The listing builds one solid part. Answer for the finished solid, in the listing's coordinates (mm). Face numbers are marked on the shaded views. A direction names the side the tool comes from. Give positions to 0.01 mm unless a question says otherwise; leave off trailing zeros. Order: outer loops, then holes, each group sorted by start corner. A loop starts at its lowest first (then second) coordinate and runs counter-clockwise, first axis right, second up. Notation, with made-up numbers: (49.25, 48) - (90.25, 48) arc R26 ccw to (90.25, 73) - close; hole circle Ø6 at (42, -1). An arc over 180 degrees is marked (long way). Answer as CSV lines item,"result". Start each with the question number.
1. Section D-D on x = 12.85 is taken. Give the vertices of the cut face in (y, z), and give its area (3 significant figures).
2. Section B-B on x = -20.35 is taken. Give the vertices of the cut face in (y, z).
3. Which of the six approach directions +Z, -Z, +X, -X, +Y, -Y give full straight-line access (tool end or side, diameter ignored) to the marked faces 1 and 2?
4. Flat-ended cylindrical pins translate along their axes: pin 1 (4 mm diameter, centred on x = 20.35, z = -6.35, fed in from -Y); pin 2 (2 mm diameter, centred on x = 10.5, y = -2, fed in from +Z); pin 3 (1.5 mm diameter, centred on y = -2, z = 7.5, fed in from +X). Find the tip coordinate at first contact, or state that the pin passes through.
5. Section C-C on z = -6.35 is taken. Give the vertices of the cut face in (x, y).
6. Consider line 1 along Y through (x, z) = (12.85, -13.55); line 2 along X through (y, z) = (0.9, 9.35); line 3 along Z through (x, y) = (15, -3.25). Determine where each line is inside the solid, lowest interval first. Write a range as [from, to].
7. Section A-A on y = -4 is taken. Give the vertices of the cut face in (x, z), and give its area (3 significant figures).
from build123d import *

# Parameters (mm, degrees)
IZIM1_W                     = 45.7
IZIM1_H                     = 24.3
Y_KSEKLIK_EKSTR_ZYON1_DEPTH = 3
IZIM2_R                     = 1.6
KES_EKSTR_ZYON1_DEPTH       = 21.8
IZIM4_W                     = 45.7
IZIM4_H                     = 2
Y_KSEKLIK_EKSTR_ZYON2_DEPTH = 10
IZIM5_R                     = 1.6
KES_EKSTR_ZYON2_DEPTH       = 4


with BuildPart() as part:
    # Çizim1 → Yükseklik-Ekstrüzyon1 (new body)
    with BuildSketch(Plane(origin=(0, 0, 0), x_dir=(1, 0, 0), z_dir=(0, 1, 0))):
        Rectangle(IZIM1_W, IZIM1_H)
    extrude(amount=Y_KSEKLIK_EKSTR_ZYON1_DEPTH)

    # Çizim2 → Kes-Ekstrüzyon1 (cut)
    with BuildSketch(Plane(origin=(0, 3, 0), x_dir=(1, 0, 0), z_dir=(0, 1, 0))):
        with Locations(Location((-20.35, -9.35, 0), (0, 0, 270))):
            Circle(IZIM2_R)
        with Locations(Location((20.35, 6.35, 0), (0, 0, 270))):
            Circle(IZIM2_R)
    extrude(amount=-KES_EKSTR_ZYON1_DEPTH, mode=Mode.SUBTRACT)

    # Çizim4 → Yükseklik-Ekstrüzyon2 (add)
    with BuildSketch(Plane(origin=(0, 3, 0), x_dir=(1, 0, 0), z_dir=(0, 1, 0))):
        with Locations((0, 13.15)):
            Rectangle(IZIM4_W, IZIM4_H)
    extrude(amount=-Y_KSEKLIK_EKSTR_ZYON2_DEPTH)

    # Çizim5 → Kes-Ekstrüzyon2 (cut)
    with BuildSketch(Plane(origin=(0, 0, -14.15), x_dir=(-1, 0, 0), z_dir=(0, 0, -1))):
        with Locations((-12.85, -4)):
            Circle(IZIM5_R)
        with Locations((12.85, -4)):
            Circle(IZIM5_R)
    extrude(amount=-KES_EKSTR_ZYON2_DEPTH, mode=Mode.SUBTRACT)


solid = part.part
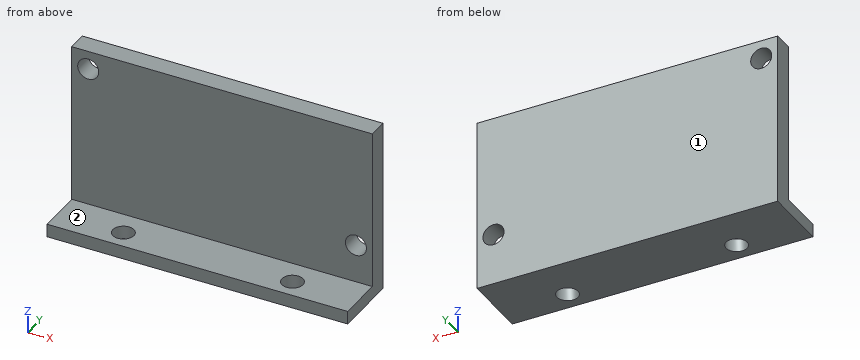
Checks:
1,outline,"(-7, -14.15) - (-5.6, -14.15) - (-5.6, -12.15) - (-7, -12.15) - close; (-2.4, -14.15) - (3, -14.15) - (3, 12.15) - (0, 12.15) - (0, -12.15) - (-2.4, -12.15) - close"
1,area,"86.5 mm²"
2,outline,"(-7, -14.15) - (3, -14.15) - (3, 7.75) - (0, 7.75) - (0, -12.15) - (-7, -12.15) - close; (0, 10.95) - (3, 10.95) - (3, 12.15) - (0, 12.15) - close"
3,face 1,"+Z, -Z, +X, -X, +Y"
3,face 2,"+Z, +X, -X, -Y"
4,pin 1,"stops at y = 0"
4,pin 2,"stops at z = -12.15"
4,pin 3,"passes through"
5,outline,"(-22.85, 0) - (18.75, 0) - (18.75, 3) - (-22.85, 3) - close; (21.95, 0) - (22.85, 0) - (22.85, 3) - (21.95, 3) - close"
6,line 1,"y = [-7, -5.6], [-2.4, 3]"
6,line 2,"x = [-22.85, -21.95], [-18.75, 22.85]"
6,line 3,"z = [-14.15, -12.15]"
7,outline,"(-22.85, -14.15) - (-14.45, -14.15) - (-14.45, -12.15) - (-22.85, -12.15) - close; (-11.25, -14.15) - (11.25, -14.15) - (11.25, -12.15) - (-11.25, -12.15) - close; (14.45, -14.15) - (22.85, -14.15) - (22.85, -12.15) - (14.45, -12.15) - close"
7,area,"78.6 mm²"
